from build123d import *

# Parameters (mm, degrees)
F1_DEPTH    = 4
F2_R        = 3
F3_T1_DEPTH = 15.252055078


# Not quite as in the source:
# - a fillet or chamfer that OpenCascade refuses, or shapes differently, is made with other operations: its cross-section is extruded or revolved along the edge and cut away or added


with BuildPart() as f1:
    # F0 (on Top) → F1 (new body)
    with BuildSketch(Plane.XY):
        with BuildLine():
            Line((8.75, 4.175), (-8.75, 4.175))
            Line((-8.75, 4.175), (-8.75, -8.825))
            Line((-8.75, -8.825), (-3.8077747211, -8.825))
            ThreePointArc((-3.8077747211, -8.825), (-4.2737752701, -4.8702772279), (-0.75, -6.725))
            ThreePointArc((-0.75, -6.725), (-1.1452772279, -7.9987752701), (-2.1922252789, -8.825))
            Line((-2.1922252789, -8.825), (2.1922252789, -8.825))
            ThreePointArc((2.1922252789, -8.825), (1.7262247299, -4.8702772279), (5.25, -6.725))
            ThreePointArc((5.25, -6.725), (4.8547227721, -7.9987752701), (3.8077747211, -8.825))
            Line((3.8077747211, -8.825), (8.75, -8.825))
            Line((8.75, -8.825), (8.75, 4.175))
        make_face()
        Polygon((-6.75, 2.175), (6.75, 2.175), (6.75, -2.175), (5.6, -2.175), (5.6, -3.075), (3.95, -3.075), (3.95, -2.175), (-3.95, -2.175), (-3.95, -3.075), (-5.6, -3.075), (-5.6, -2.175), (-6.75, -2.175), align=None, mode=Mode.SUBTRACT)
    extrude(amount=F1_DEPTH)

    # F2
    f2_edges = [f1.edges().sort_by_distance(p)[0] for p in [
        (-8.75, 4.175, 2),
        (-8.75, -8.825, 2),
        (8.75, -8.825, 2),
        (8.75, 4.175, 2),
    ]]
    fillet(f2_edges, radius=F2_R)

    # F3: fillet of radius 1 on 2 edges, made by hand

    # F3_s2 → F3_t1 (cut)
    with BuildSketch(Plane.XY.offset(-5.626027539)):
        with BuildLine():
            ThreePointArc((0.88279449, -7.4865384615), (0.7598795231, -8.4001254044), (-0.0581857367, -8.825))
            Line((-0.0581857367, -8.825), (2.1922252789, -8.825))
            ThreePointArc((2.1922252789, -8.825), (1.3916632316, -8.2984525222), (0.88279449, -7.4865384615))
        make_face()
        with BuildLine():
            ThreePointArc((0.0581857367, -8.825), (-0.7598795231, -8.4001254044), (-0.88279449, -7.4865384615))
            ThreePointArc((-0.88279449, -7.4865384615), (-1.3916632316, -8.2984525222), (-2.1922252789, -8.825))
            Line((-2.1922252789, -8.825), (0.0581857367, -8.825))
        make_face()
    extrude(amount=F3_T1_DEPTH, mode=Mode.SUBTRACT)


solid = f1.part
Check sheet for the modelled part. Datum: model origin and axes. Units: mm. A direction names the side the tool comes from. Round coordinates to 2 decimals unless told otherwise and drop trailing zeros. Order: outer loops, then holes, each group sorted by start corner. A loop starts at its lowest first (then second) coordinate and runs counter-clockwise, first axis right, second up.
(1) Draft check along X on faces 1 (the flat face through (-5, -3.075, 2)), 2 (the cylindrical face through (-7.85, 3.32, 2.03)), 3 (the flat face through (-5, -8.825, 2)). Enter one of: pulls with the +X half, pulls with the -X half, needs draft (parallel to the pull), parting line crosses it, or undercut.
(2) Cross-section at B-B, the plane y = -0.75. Enter the section's corners in (x, z), and give its area (3 significant figures).
(3) Scan lines: probe 1 along X at (y, z) = (-3, 0.7); probe 2 along Y at (x, z) = (-5.5, 2.6) (3 decimals); probe 3 along Y at (x, z) = (3, 2.75) (3 decimals). Record each from-to range of solid material in increasing order.
(4) Cross-section at D-D, the plane z = 3.35. Enter the section's corners in (x, y) (3 decimals), and give its area (3 significant figures).
(5) Access from +Z, -Z, +X, -X, +Y, -Y to the whole of each face (thin tool, end or side, straight path). Record for faces 4 (the flat face through (0, 4.175, 2)), 5 (the flat face through (0, -2.175, 2)).
(6) Cross-section at A-A, the plane x = -3. Enter the section's corners in (y, z) (3 decimals).
(7) Cross-section at C-C, the plane y = -6.5. Enter the section's corners in (x, z), and give its area (3 significant figures).
Check sheet entries:
1. face 1: undercut
1. face 2: pulls with the -X half
1. face 3: needs draft
2. outline: (-8.75, 0) - (-6.75, 0) - (-6.75, 4) - (-8.75, 4) - close; (6.75, 0) - (8.75, 0) - (8.75, 4) - (6.75, 4) - close
2. area: 16.0 mm2
3. probe 1: x = -8.75 to -5.6, -3.95 to 3.95, 5.6 to 8.75
3. probe 2: y = -8.825 to -3.075, 2.175 to 4.175
3. probe 3: y = -4.475 to -2.175, 2.175 to 4.175
4. outline: (-8.75, -5.825) arc R3 ccw to (-5.75, -8.825) - (-3.808, -8.825) arc R2.25 cw (long way) to (-0.883, -7.487) arc R1 ccw to (0, -8.823) arc R1 ccw to (0.883, -7.487) arc R2.25 cw (long way) to (3.808, -8.825) - (5.75, -8.825) arc R3 ccw to (8.75, -5.825) - (8.75, 1.175) arc R3 ccw to (5.75, 4.175) - (-5.75, 4.175) arc R3 ccw to (-8.75, 1.175) - close; hole (-6.75, -2.175) - (-5.6, -2.175) - (-5.6, -3.075) - (-3.95, -3.075) - (-3.95, -2.175) - (3.95, -2.175) - (3.95, -3.075) - (5.6, -3.075) - (5.6, -2.175) - (6.75, -2.175) - (6.75, 2.175) - (-6.75, 2.175) - close
4. area: 125 mm2
5. face 4: +Z, -Z, +X, -X, +Y
5. face 5: +Z, -Z
6. outline: (-4.475, 0) - (-2.175, 0) - (-2.175, 4) - (-4.475, 4) - close; (2.175, 0) - (4.175, 0) - (4.175, 4) - (2.175, 4) - close
7. outline: (-8.67, 0) - (-5.24, 0) - (-5.24, 4) - (-8.67, 4) - close; (-0.76, 0) - (0.76, 0) - (0.76, 4) - (-0.76, 4) - close; (5.24, 0) - (8.67, 0) - (8.67, 4) - (5.24, 4) - close
7. area: 33.6 mm2
